from build123d import *

# Parameters (mm, degrees)
BOSS_EXTRUDE1_DEPTH                               = 5.715
SKETCH1_W                                         = 202
SKETCH1_H                                         = 222
CUT_EXTRUDE1_DEPTH                                = 6.715
CSK_FOR_6_FLAT_HEAD_SOCKET_CAP_SCREW1_D           = 3.7973
CSK_FOR_6_FLAT_HEAD_SOCKET_CAP_SCREW1_DEPTH       = 20
CSK_FOR_6_FLAT_HEAD_SOCKET_CAP_SCREW1_CSINK_D     = 7.7978
CSK_FOR_6_FLAT_HEAD_SOCKET_CAP_SCREW1_CSINK_ANGLE = 82
CSK_FOR_6_FLAT_HEAD_SOCKET_CAP_SCREW1_TIP         = 1.140824014


with BuildPart() as part:
    # Model → Boss-Extrude1 (new body)
    with BuildSketch(Plane.XY):
        Polygon((1024.07974, 23.2006394), (1029.90396, 23.2006394), (1029.90396, 28.91536), (1041.33396, 28.91536), (1041.33396, 23.2006394), (1052.76396, 23.2006394), (1052.76396, 28.91536), (1064.19396, 28.91536), (1064.19396, 23.2006394), (1075.62396, 23.2006394), (1075.62396, 28.91536), (1087.05396, 28.91536), (1087.05396, 23.2006394), (1098.48396, 23.2006394), (1098.48396, 28.91536), (1109.91396, 28.91536), (1109.91396, 23.2006394), (1121.34396, 23.2006394), (1121.34396, 28.91536), (1132.77396, 28.91536), (1132.77396, 23.2006394), (1144.20396, 23.2006394), (1144.20396, 28.91536), (1155.63396, 28.91536), (1155.63396, 23.2006394), (1167.06396, 23.2006394), (1167.06396, 28.91536), (1178.49396, 28.91536), (1178.49396, 23.2006394), (1189.92396, 23.2006394), (1189.92396, 28.91536), (1201.35396, 28.91536), (1201.35396, 23.2006394), (1212.78396, 23.2006394), (1212.78396, 28.91536), (1224.21396, 28.91536), (1224.21396, 23.2006394), (1235.75318, 23.2006394), (1235.75318, 279.63114), (1224.21396, 279.63114), (1224.21396, 273.91614), (1212.78396, 273.91614), (1212.78396, 279.63114), (1201.35396, 279.63114), (1201.35396, 273.91614), (1189.92396, 273.91614), (1189.92396, 279.63114), (1178.49396, 279.63114), (1178.49396, 273.91614), (1167.06396, 273.91614), (1167.06396, 279.63114), (1155.63396, 279.63114), (1155.63396, 273.91614), (1144.20396, 273.91614), (1144.20396, 279.63114), (1132.77396, 279.63114), (1132.77396, 273.91614), (1121.34396, 273.91614), (1121.34396, 279.63114), (1109.91396, 279.63114), (1109.91396, 273.91614), (1098.48396, 273.91614), (1098.48396, 279.63114), (1087.05396, 279.63114), (1087.05396, 273.91614), (1075.62396, 273.91614), (1075.62396, 279.63114), (1064.19396, 279.63114), (1064.19396, 273.91614), (1052.76396, 273.91614), (1052.76396, 279.63114), (1041.33396, 279.63114), (1041.33396, 273.91614), (1029.90396, 273.91614), (1029.90396, 279.63114), (1024.07974, 279.63114), align=None)
    extrude(amount=BOSS_EXTRUDE1_DEPTH)

    # Sketch1 → Cut-Extrude1 (cut, through all)
    with BuildSketch(Plane(origin=(0, 0, 0), x_dir=(-1, 0, 0), z_dir=(0, 0, -1))):
        with Locations((-1129.03818, 151.41575)):
            Rectangle(SKETCH1_W, SKETCH1_H)
    extrude(amount=-CUT_EXTRUDE1_DEPTH, mode=Mode.SUBTRACT)

    # CSK for #6 Flat Head Socket Cap Screw1
    with Locations(Plane(origin=(1095.03845, 151.41575, 0), x_dir=(-1, 0, 0), z_dir=(0, 0, -1))):
        with Locations((-119.24973, 115), (-33.99973, 115), (51.25027, 115), (51.25027, -115), (-33.99973, -115), (-119.24973, -115)):
            CounterSinkHole(CSK_FOR_6_FLAT_HEAD_SOCKET_CAP_SCREW1_D / 2, CSK_FOR_6_FLAT_HEAD_SOCKET_CAP_SCREW1_CSINK_D / 2, depth=CSK_FOR_6_FLAT_HEAD_SOCKET_CAP_SCREW1_DEPTH, counter_sink_angle=CSK_FOR_6_FLAT_HEAD_SOCKET_CAP_SCREW1_CSINK_ANGLE)
            with Locations((0, 0, -(CSK_FOR_6_FLAT_HEAD_SOCKET_CAP_SCREW1_DEPTH + CSK_FOR_6_FLAT_HEAD_SOCKET_CAP_SCREW1_TIP / 2))):  # 118° drill point
                Cone(0, CSK_FOR_6_FLAT_HEAD_SOCKET_CAP_SCREW1_D / 2, CSK_FOR_6_FLAT_HEAD_SOCKET_CAP_SCREW1_TIP, mode=Mode.SUBTRACT)


solid = part.part
Geometry check sheet. Reference: the model listing, model coordinates, mm. A direction names the side the tool comes from. Give positions to 0.01 mm unless a question says otherwise; leave off trailing zeros. Loops run counter-clockwise (first coordinate to the right, second up) from the corner with the lowest first, then second, coordinate; pieces in that order, holes last. Notation, with made-up numbers: (-20.5, 87) -> (25.5, 87) arc R12 cw to (25.5, 103) -> close; hole circle Ø10 at (72, 52.25). An arc over 180 degrees is marked (long way). Answer in a Markdown table with one row per item. Add a question column.
1) Gauge pin test, flat end, axial feed: P1, Ø1.7, axis at x = 1147.5, z = 2.5, coming from the -Y side. Record the tip position at first contact, or that the pin passes through.
2) Cross-section at B-B on y = 114.5. Record the boundary of the cut face in (x, z) (3 decimals).
3) Cross-section at C-C on z = 4.2. State how many separate pieces and enclosed holes the cut face has, and give its area (3 significant figures).
4) Set-up check for faces 4 (the face through (1150, 28.915, 3)), 5 (the face through (1184, 279.631, 3)), 6 (the face through (1052.764, 277, 3)): record each of +Z, -Z, +X, -X, +Y, -Y from which the full face is reachable in a straight line by a thin tool's end or side.
5) Cross-section at A-A on x = 1094. Record the boundary of the cut face in (y, z) (3 decimals).
6) Material ranges on probe 1 along Y at (x, z) = (1082, 2.9); probe 2 along Y at (x, z) = (1090, 2.6); probe 3 along X at (y, z) = (183, 0.45), recorded low to high. Write a range as from..to.
7) Draft check along X on faces 1 (the face through (1047, 23.201, 3)), 2 (the face through (1230.038, 150, 3)), 3 (the face through (1041.334, 26, 3)). Enter one of: pulls with the +X half, pulls with the -X half, needs draft (parallel to the pull), parting line crosses it, or undercut.
Outcome:
| question | item | result |
|---|---|---|
| 1 | P1 | stops at y = 28.92 |
| 2 | outline | (1024.08, 0) -> (1028.038, 0) -> (1028.038, 5.715) -> (1024.08, 5.715) -> close; (1230.038, 0) -> (1235.753, 0) -> (1235.753, 5.715) -> (1230.038, 5.715) -> close |
| 3 | separate pieces | 1 |
| 3 | enclosed holes | 7 |
| 3 | area | 8,190 mm^2 |
| 4 | face 4 | +Z, -Z, -Y |
| 4 | face 5 | +Z, -Z, +X, -X, +Y |
| 4 | face 6 | +Z, -Z, +Y |
| 5 | outline | (23.201, 0) -> (40.416, 0) -> (40.416, 5.715) -> (23.201, 5.715) -> close; (262.416, 0) -> (279.631, 0) -> (279.631, 5.715) -> (262.416, 5.715) -> close |
| 6 | probe 1 | y = 28.92..40.42, 262.42..273.92 |
| 6 | probe 2 | y = 23.2..40.42, 262.42..279.63 |
| 6 | probe 3 | x = 1024.08..1028.04, 1230.04..1235.75 |
| 7 | face 1 | needs draft |
| 7 | face 2 | undercut |
| 7 | face 3 | undercut |
